from build123d import *

# Parameters (mm, degrees)
EXTRUDE_1_DEPTH = 30
EXTRUDE_2_DEPTH = 6


with BuildPart() as part:
    # 草图1 → 凸台-拉伸1 (new body)
    with BuildSketch(Plane.XY):
        with BuildLine():
            Line((0, 6.25), (0, 11.25))
            ThreePointArc((0, 11.25), (-11.25, 0), (0, -11.25))
            Line((0, -11.25), (0, -6.25))
            ThreePointArc((0, -6.25), (-6.25, 0), (0, 6.25))
        make_face()
    extrude(amount=EXTRUDE_1_DEPTH)

    # 草图2 → 凸台-拉伸2 (add)
    with BuildSketch(Plane.XY.offset(30)):
        with BuildLine():
            Line((0, 6.25), (0, 11.25))
            ThreePointArc((0, 11.25), (-6.708203932, 9.031195934), (-10.770329614, 3.25))
            Line((-10.770329614, 3.25), (-5.338539126, 3.25))
            ThreePointArc((-5.338539126, 3.25), (-3.061862178, 5.448623679), (0, 6.25))
        make_face()
        with BuildLine():
            Line((11.25, 3.25), (11.25, 11.25))
            Line((11.25, 11.25), (0, 11.25))
            Line((0, 11.25), (0, 6.25))
            ThreePointArc((0, 6.25), (-3.061862178, 5.448623679), (-5.338539126, 3.25))
            Line((-5.338539126, 3.25), (11.25, 3.25))
        make_face()
        with BuildLine():
            ThreePointArc((0, -6.25), (-3.061862178, -5.448623679), (-5.338539126, -3.25))
            Line((-5.338539126, -3.25), (-10.770329614, -3.25))
            ThreePointArc((-10.770329614, -3.25), (-6.708203932, -9.031195934), (0, -11.25))
            Line((0, -11.25), (0, -6.25))
        make_face()
        with BuildLine():
            Line((11.25, -11.25), (11.25, -3.25))
            Line((11.25, -3.25), (-5.338539126, -3.25))
            ThreePointArc((-5.338539126, -3.25), (-3.061862178, -5.448623679), (0, -6.25))
            Line((0, -6.25), (0, -11.25))
            Line((0, -11.25), (11.25, -11.25))
        make_face()
    extrude(amount=EXTRUDE_2_DEPTH)


solid = part.part
Can you work these out from the model? Positions are in its coordinate system, mm. A direction names the side the tool comes from. Coordinates: 2 decimals unless noted, no trailing zeros. Write each loop counter-clockwise with the first axis right and the second up, starting at its lowest first coordinate (ties: lowest second). Pieces come first, ordered by that corner, then holes.
Q1. Please list where these lines run through material, in increasing order: L1, parallel to Z at x = 4.75, y = 6; L2, parallel to Y at x = -4.5, z = 17; L3, parallel to Z at x = -8.25, y = -0.5.
Results found:
L1: z = 30 to 36
L2: y = -10.31 to -4.34, 4.34 to 10.31
L3: z = 0 to 30
Q2. Imagine slicing it at D-D, the plane y = 0. List the corners of the cut face in (x, z) for me, plus the area to 3 significant figures.
Results found:
outline: (-11.25, 0) - (-6.25, 0) - (-6.25, 30) - (-11.25, 30) - close
area: 150 mm2
Q3. Imagine slicing it at C-C, the plane x = -9. List the corners of the cut face in (y, z) for me.
Results found:
outline: (-6.75, 0) - (6.75, 0) - (6.75, 36) - (3.25, 36) - (3.25, 30) - (-3.25, 30) - (-3.25, 36) - (-6.75, 36) - close
Q4. For P1, Ø8, axis at y = 0.5, z = 18.5, coming from the +X side; P2, Ø5, axis at y = -7.5, z = 23, coming from the +X side; P3, Ø9, axis at x = 5.5, y = -8, coming from the -Z side, each with a flat end and sliding along its axis, tell me the tip position at first contact or that it passes through.
Results found:
P1: stops at x = -4.34
P2: stops at x = 0
P3: stops at z = 30
Q5. Which directions (+Z, -Z, +X, -X, +Y, -Y) give clear straight access to the entire face, cutting with the end or side of a thin tool? Please do faces 5 (the face through (0, 7, 36)), 6 (the face through (0, 3.25, 33)), 7 (the face through (-6.25, -0.14, 14.79)), 8 (the face through (0, -9, 15)).
Results found:
face 5: +Z, +X, -X, +Y, -Y
face 6: +Z, +X, -X
face 7: -Z, +X
face 8: -Z, +X, +Y, -Y
Q6. Imagine slicing it at A-A, the plane x = 1.5. List the corners of the cut face in (y, z) for me.
Results found:
outline: (-11.25, 30) - (-3.25, 30) - (-3.25, 36) - (-11.25, 36) - close; (3.25, 30) - (11.25, 30) - (11.25, 36) - (3.25, 36) - close
Q7. Imagine slicing it at B-B, the plane z = 33. List the corners of the cut face in (x, y) for me.
Results found:
outline: (-10.77, -3.25) arc R11.25 ccw to (0, -11.25) - (11.25, -11.25) - (11.25, -3.25) - close; (-10.77, 3.25) - (11.25, 3.25) - (11.25, 11.25) - (0, 11.25) arc R11.25 ccw to start
Q8. If we mould it in two halves opening along Y, with no side actions, what happens to faces 1 (the face through (6, 11.25, 33)), 2 (the face through (6, -11.25, 33)), 3 (the face through (-8, 0, 30)), 4 (the face through (0, 9, 15))? For each: +Y half, -Y half, draft (parallel to the pull), parting line (faces both ways), or undercut.
Results found:
face 1: +Y half
face 2: -Y half
face 3: undercut
face 4: draft
